Check sheet for the modelled part. Datum: model origin and axes. Units: mm. Round coordinates to 2 decimals unless told otherwise and drop trailing zeros. Loops run counter-clockwise (first coordinate to the right, second up) from the corner with the lowest first, then second, coordinate; pieces in that order, holes last. Notation, with made-up numbers: (7, -6.5) -> (54, -6.5) arc R20 ccw to (54, 29.5) -> close; hole circle Ø1 at (-31, 64). An arc over 180 degrees is marked (long way). Use one line per item in the form item = value. Start each with the question number.
(1) Sectioned sample at C-C (x = 14). Record the cut outline in (y, z), and give its area (3 significant figures).
(2) Sectioned sample at A-A (y = -4.5). Record the cut outline in (x, z).
(3) Go/stop test with a flat-tipped pin: pin 1 (4 mm diameter, centred on x = 43.57, y = -42.81, fed in from -Z). Record where the tip stops, or that it passes through.
(4) Material ranges on probe 1 along X at (y, z) = (-15, 4.65); probe 2 along Y at (x, z) = (33, 4.15) (3 decimals); probe 3 along Y at (x, z) = (-17, 1.5), recorded low to high. Write a range as [from, to].
(5) Sectioned sample at D-D (z = 1.3). State how many separate pieces and enclosed holes the cut face has, and give its area (3 significant figures).
(6) Sectioned sample at B-B (x = -13.5). Record the cut outline in (y, z).
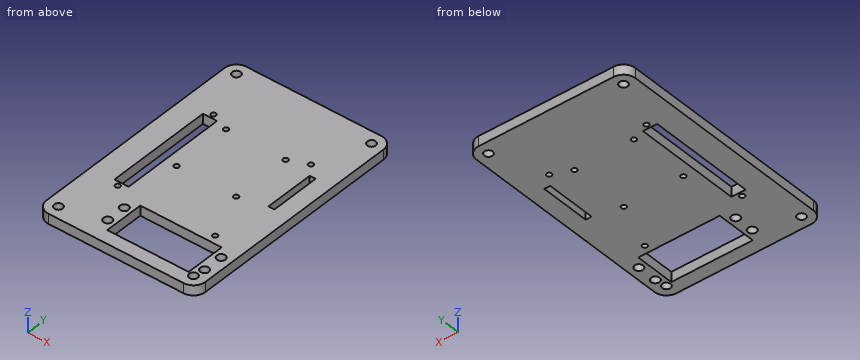
from build123d import *

# Parameters (mm, degrees)
IZIM1_W                              = 80
IZIM1_H                              = 100
Y_KSEKLIK_EKSTR_ZYON1_DEPTH          = 5
IZIM2_R                              = 1.25
IZIM2_R_2                            = 1.286520495
KES_EKSTR_ZYON1_DEPTH                = 10
M4_HELISARMAL_I_IN_Z_VANA_MATKAB_1_D = 4.2
RADYUS1_R                            = 6
RADYUS2_R                            = 6
RADYUS3_R                            = 6
RADYUS4_R                            = 6
IZIM4_W                              = 3
IZIM4_H                              = 25
IZIM4_R                              = 1.25
IZIM4_R_2                            = 1.255794896
KES_EKSTR_ZYON2_DEPTH                = 50
IZIM5_W                              = 7.124534101
IZIM5_H                              = 53.617419338
KES_EKSTR_ZYON3_DEPTH                = 50
IZIM6_R                              = 2.6
IZIM6_R_2                            = 2.15
IZIM6_R_3                            = 2.1
Y_KSEKLIK_EKSTR_ZYON2_DEPTH          = 5
IZIM7_R                              = 2.15
KES_EKSTR_ZYON4_DEPTH                = 5
KES_EKSTR_ZYON5_DEPTH                = 5


with BuildPart() as part:
    # Çizim1 → Yükseklik-Ekstrüzyon1 (new body)
    with BuildSketch(Plane.XY):
        with Locations((8.667082878, 5.369127517)):
            Rectangle(IZIM1_W, IZIM1_H)
    extrude(amount=Y_KSEKLIK_EKSTR_ZYON1_DEPTH)

    # Çizim2 → Kes-Ekstrüzyon1 (cut)
    with BuildSketch(Plane(origin=(0, 0, 0), x_dir=(-1, 0, 0), z_dir=(0, 0, -1))):
        with Locations((15.957451223, 24.185733017)):
            Circle(IZIM2_R)
        with Locations((-33.042548777, 24.185733017)):
            Circle(IZIM2_R)
        with Locations((-33.042548777, -33.814266983)):
            Circle(IZIM2_R)
        with Locations((15.957451223, -33.814266983)):
            Circle(IZIM2_R_2)
    extrude(amount=-KES_EKSTR_ZYON1_DEPTH, mode=Mode.SUBTRACT)

    # M4 Helisarmal için Zıvana matkabı1 (through all)
    with Locations(Plane(origin=(-25.332917122, -38.630872483, 0), x_dir=(-1, 0, 0), z_dir=(0, 0, -1))):
        with Locations((0, 0), (-68, 0), (0, 88), (-68, 88)):
            Hole(M4_HELISARMAL_I_IN_Z_VANA_MATKAB_1_D / 2)

    # Radyus1
    radyus1_edges = [part.edges().sort_by_distance(p)[0] for p in [
        (-31.332917122, 55.369127517, 2.5),
    ]]
    fillet(radyus1_edges, radius=RADYUS1_R)

    # Radyus2
    radyus2_edges = [part.edges().sort_by_distance(p)[0] for p in [
        (-31.332917122, -44.630872483, 2.5),
    ]]
    fillet(radyus2_edges, radius=RADYUS2_R)

    # Radyus3
    radyus3_edges = [part.edges().sort_by_distance(p)[0] for p in [
        (48.667082878, -44.630872483, 2.5),
    ]]
    fillet(radyus3_edges, radius=RADYUS3_R)

    # Radyus4
    radyus4_edges = [part.edges().sort_by_distance(p)[0] for p in [
        (48.667082878, 55.369127517, 2.5),
    ]]
    fillet(radyus4_edges, radius=RADYUS4_R)

    # Çizim4 → Kes-Ekstrüzyon2 (cut)
    with BuildSketch(Plane.XY.offset(5)):
        with Locations((38.703217921, 5.985733017)):
            Rectangle(IZIM4_W, IZIM4_H)
        with Locations((23.667082878, -9.814266983)):
            Circle(IZIM4_R)
        with Locations((23.667082878, 20.185733017)):
            Circle(IZIM4_R_2)
        with Locations((-6.332917122, 20.185733017)):
            Circle(IZIM4_R)
        with Locations((-6.332917122, -9.814266983)):
            Circle(IZIM4_R)
    extrude(amount=-KES_EKSTR_ZYON2_DEPTH, mode=Mode.SUBTRACT)

    # Çizim5 → Kes-Ekstrüzyon3 (cut)
    with BuildSketch(Plane(origin=(0, 0, 0), x_dir=(-1, 0, 0), z_dir=(0, 0, -1))):
        with Locations((15.895184173, -4.826044253)):
            Rectangle(IZIM5_W, IZIM5_H)
    extrude(amount=-KES_EKSTR_ZYON3_DEPTH, mode=Mode.SUBTRACT)

    # Çizim6 → Yükseklik-Ekstrüzyon2 (add)
    # profile 1 of 3: a face of its own
    with BuildSketch(Plane.XY.offset(5)):
        with Locations((-25.332917122, -38.630872483)):
            Circle(IZIM6_R)
    # profile 2 of 3: a face of its own
    with BuildSketch(Plane.XY.offset(5)):
        with Locations((42.667082878, -38.630872483)):
            Circle(IZIM6_R)
    # profile 3 of 3: a face of its own
    with BuildSketch(Plane.XY.offset(5)):
        with BuildLine():
            Line((-31.332917122, -38.630872483), (48.667082878, -38.630872483))
            Line((48.667082878, -38.630872483), (48.667082878, -58.482911504))
            ThreePointArc((48.667082878, -58.482911504), (46.909723565, -62.725552191), (42.667082878, -64.482911504))
            Line((42.667082878, -64.482911504), (-25.332917122, -64.482911504))
            ThreePointArc((-25.332917122, -64.482911504), (-29.575557809, -62.725552191), (-31.332917122, -58.482911504))
            Line((-31.332917122, -58.482911504), (-31.332917122, -38.630872483))
        make_face()
        with Locations((-5.232917122, -52.814266983)):
            Circle(IZIM6_R_2, mode=Mode.SUBTRACT)
        with Locations((-5.232917122, -42.814266983)):
            Circle(IZIM6_R_2, mode=Mode.SUBTRACT)
        with Locations((43.567082878, -42.814266983)):
            Circle(IZIM6_R_2, mode=Mode.SUBTRACT)
        with Locations((43.567082878, -52.814266983)):
            Circle(IZIM6_R_2, mode=Mode.SUBTRACT)
        with Locations((-25.332917122, -58.482911504)):
            Circle(IZIM6_R_3, mode=Mode.SUBTRACT)
        with Locations((42.667082878, -58.482911504)):
            Circle(IZIM6_R_3, mode=Mode.SUBTRACT)
    extrude(amount=-Y_KSEKLIK_EKSTR_ZYON2_DEPTH)

    # Çizim7 → Kes-Ekstrüzyon4 (cut)
    with BuildSketch(Plane.XY.offset(5)):
        with Locations((43.567082878, -42.814266983)):
            Circle(IZIM7_R)
        with Locations((-5.232917122, -42.814266983)):
            Circle(IZIM7_R)
    extrude(amount=-KES_EKSTR_ZYON4_DEPTH, mode=Mode.SUBTRACT)

    # Çizim8 → Kes-Ekstrüzyon5 (cut)
    with BuildSketch(Plane.XY.offset(5)):
        Polygon((-1.332917122, -37.814266983), (-1.332917122, -38.614266983), (-1.332917122, -57.814266983), (39.667082878, -57.814266983), (39.667082878, -37.814266983), align=None)
    extrude(amount=-KES_EKSTR_ZYON5_DEPTH, mode=Mode.SUBTRACT)


solid = part.part
Checks:
q1.outline = (-64.48, 0) -> (-57.81, 0) -> (-57.81, 5) -> (-64.48, 5) -> close; (-37.81, 0) -> (55.37, 0) -> (55.37, 5) -> (-37.81, 5) -> close
q1.area = 499 mm2
q2.outline = (-31.33, 0) -> (-19.46, 0) -> (-19.46, 5) -> (-31.33, 5) -> close; (-12.33, 0) -> (37.2, 0) -> (37.2, 5) -> (-12.33, 5) -> close; (40.2, 0) -> (48.67, 0) -> (48.67, 5) -> (40.2, 5) -> close
q3.pin_1 = through
q4.probe_1 = [-31.33, -19.46], [-12.33, 48.67]
q4.probe_2 = [-64.483, -57.814], [-37.814, -35.064], [-32.565, 22.936], [25.435, 55.369]
q4.probe_3 = [-64.48, -34.57], [-33.06, -31.63], [21.98, 23.5], [24.88, 55.37]
q5.separate_pieces = 1
q5.enclosed_holes = 19
q5.area = 8,130 mm2
q6.outline = (-64.48, 0) -> (-31.63, 0) -> (-31.63, 5) -> (-64.48, 5) -> close; (21.98, 0) -> (55.37, 0) -> (55.37, 5) -> (21.98, 5) -> close
